Here's how the part is built. I have some questions about the finished solid (model axes, mm). Coordinates: 2 decimals unless noted, no trailing zeros. Write each loop counter-clockwise with the first axis right and the second up, starting at its lowest first coordinate (ties: lowest second). Pieces come first, ordered by that corner, then holes. Notation, with made-up numbers: M 15,89.5 L 27,89.5 A7 cw 27,96.5 Z; hole C 24.25,-26 d11. An arc over 180 degrees is marked long. Use one line per item in the form item = value. Start each with the question number.
1. I want a section at A-A, the plane z = 125.5. List the corners of the cut face in (x, y) for me.
2. Please list where these lines run through material, in increasing order: line 1 along X through (y, z) = (7.25, 121); line 2 along Z through (x, y) = (26, 8.25); line 3 along X through (y, z) = (8.75, 178). Write a range as [from, to].
3. I'm going to push flat-ended pins straight in: pin 1 Ø3 at (y, z) = (4, 230.5) entering from -X; pin 2 Ø6 at (x, z) = (83.5, 111) entering from -Y; pin 3 Ø3 at (x, y) = (201.5, 5.5) entering from -Z. Where does each tip first touch, or does it pass through?
4. I want a section at B-B, the plane z = 212. List the corners of the cut face in (x, y) for me.
5. I want a section at C-C, the plane y = 2. Count the separate pieces of the cut face and the enclosed holes in it, plus the area to 3 significant figures.
from build123d import *

# Parameters (mm, degrees)
SKETCH_1_R      = 3.519137415
SKETCH_1_R_2    = 4.021871331
SKETCH_1_R_3    = 4.053170413
SKETCH_1_R_4    = 3.845688718
SKETCH_1_R_5    = 4
EXTRUDE_1_DEPTH = 10


with BuildPart() as part:
    # 草图1 → 凸台-拉伸1 (new body)
    with BuildSketch(Plane(origin=(0, 0, 0), x_dir=(1, 0, 0), z_dir=(0, 1, 0))):
        Polygon((0, -50), (75, -50), (75, 0), (175, 0), (175, -50), (250, -50), (250, -200), (175, -200), (175, -250), (75, -250), (75, -200), (0, -200), align=None)
        with Locations(Location((140.533556543, -125.014564911, 0), (0, 0, 270))):
            Circle(SKETCH_1_R, mode=Mode.SUBTRACT)
        with Locations(Location((121.008156214, -98.872401259, 0), (0, 0, 270))):
            Circle(SKETCH_1_R_2, mode=Mode.SUBTRACT)
        with Locations(Location((121.008156214, -150.151260731, 0), (0, 0, 270))):
            Circle(SKETCH_1_R_3, mode=Mode.SUBTRACT)
        with Locations(Location((99.599362347, -125.014564911, 0), (0, 0, 270))):
            Circle(SKETCH_1_R_4, mode=Mode.SUBTRACT)
        with Locations(Location((85.515139111, -8.883030225, 0), (0, 0, 270))):
            Circle(SKETCH_1_R_5, mode=Mode.SUBTRACT)
        with Locations(Location((85.515139111, -30.50058863, 0), (0, 0, 270))):
            Circle(SKETCH_1_R_5, mode=Mode.SUBTRACT)
        with Locations(Location((107.349135631, -8.883030225, 0), (0, 0, 270))):
            Circle(SKETCH_1_R_5, mode=Mode.SUBTRACT)
        with Locations(Location((107.349135631, -30.50058863, 0), (0, 0, 270))):
            Circle(SKETCH_1_R_5, mode=Mode.SUBTRACT)
        with Locations(Location((146.396218991, -8.883030225, 0), (0, 0, 270))):
            Circle(SKETCH_1_R_5, mode=Mode.SUBTRACT)
        with Locations(Location((166.756942605, -8.883030225, 0), (0, 0, 270))):
            Circle(SKETCH_1_R_5, mode=Mode.SUBTRACT)
        with Locations(Location((146.396218991, -30.50058863, 0), (0, 0, 270))):
            Circle(SKETCH_1_R_5, mode=Mode.SUBTRACT)
        with Locations(Location((166.756942605, -30.50058863, 0), (0, 0, 270))):
            Circle(SKETCH_1_R_5, mode=Mode.SUBTRACT)
        with Locations(Location((85.515139111, -237.626962183, 0), (0, 0, 270))):
            Circle(SKETCH_1_R_5, mode=Mode.SUBTRACT)
        with Locations(Location((85.515139111, -212.99300028, 0), (0, 0, 270))):
            Circle(SKETCH_1_R_5, mode=Mode.SUBTRACT)
        with Locations(Location((107.217902356, -212.99300028, 0), (0, 0, 270))):
            Circle(SKETCH_1_R_5, mode=Mode.SUBTRACT)
        with Locations(Location((107.217902356, -237.626962183, 0), (0, 0, 270))):
            Circle(SKETCH_1_R_5, mode=Mode.SUBTRACT)
        with Locations(Location((162.537022604, -212.99300028, 0), (0, 0, 270))):
            Circle(SKETCH_1_R_5, mode=Mode.SUBTRACT)
        with Locations(Location((162.537022604, -237.626962183, 0), (0, 0, 270))):
            Circle(SKETCH_1_R_5, mode=Mode.SUBTRACT)
        with Locations(Location((140.533556543, -212.99300028, 0), (0, 0, 270))):
            Circle(SKETCH_1_R_5, mode=Mode.SUBTRACT)
        with Locations(Location((140.533556543, -237.626962183, 0), (0, 0, 270))):
            Circle(SKETCH_1_R_5, mode=Mode.SUBTRACT)
        with Locations(Location((9.903960691, -59.156421864, 0), (0, 0, 270))):
            Circle(SKETCH_1_R_5, mode=Mode.SUBTRACT)
        with Locations(Location((242.167030064, -59.156421864, 0), (0, 0, 270))):
            Circle(SKETCH_1_R_5, mode=Mode.SUBTRACT)
        with Locations(Location((242.167030064, -187.85630446, 0), (0, 0, 270))):
            Circle(SKETCH_1_R_5, mode=Mode.SUBTRACT)
        with Locations(Location((204.964720251, -59.156421864, 0), (0, 0, 270))):
            Circle(SKETCH_1_R_5, mode=Mode.SUBTRACT)
        with Locations(Location((204.964720251, -187.85630446, 0), (0, 0, 270))):
            Circle(SKETCH_1_R_5, mode=Mode.SUBTRACT)
        with Locations(Location((9.903960691, -187.85630446, 0), (0, 0, 270))):
            Circle(SKETCH_1_R_5, mode=Mode.SUBTRACT)
        with Locations(Location((43.587133089, -59.156421864, 0), (0, 0, 270))):
            Circle(SKETCH_1_R_5, mode=Mode.SUBTRACT)
        with Locations(Location((43.587133089, -187.85630446, 0), (0, 0, 270))):
            Circle(SKETCH_1_R_5, mode=Mode.SUBTRACT)
        with Locations(Location((69.226562825, -59.156421864, 0), (0, 0, 270))):
            Circle(SKETCH_1_R_5, mode=Mode.SUBTRACT)
        with Locations(Location((69.226562825, -187.85630446, 0), (0, 0, 270))):
            Circle(SKETCH_1_R_5, mode=Mode.SUBTRACT)
        with Locations(Location((179.828024432, -59.156421864, 0), (0, 0, 270))):
            Circle(SKETCH_1_R_5, mode=Mode.SUBTRACT)
        with Locations(Location((179.828024432, -187.85630446, 0), (0, 0, 270))):
            Circle(SKETCH_1_R_5, mode=Mode.SUBTRACT)
        with BuildLine():
            Line((31.521519096, -110.938015252), (31.521519096, -139.09111457))
            ThreePointArc((31.521519096, -139.09111457), (26.494179932, -144.118453734), (21.466840768, -139.09111457))
            Line((21.466840768, -139.09111457), (21.466840768, -110.938015252))
            ThreePointArc((21.466840768, -110.938015252), (26.494179932, -105.910676088), (31.521519096, -110.938015252))
        make_face(mode=Mode.SUBTRACT)
        with BuildLine():
            Line((31.521519096, -59.156421864), (31.521519096, -88.314989015))
            ThreePointArc((31.521519096, -88.314989015), (26.494179932, -93.342328179), (21.466840768, -88.314989015))
            Line((21.466840768, -88.314989015), (21.466840768, -59.156421864))
            ThreePointArc((21.466840768, -59.156421864), (26.494179932, -54.1290827), (31.521519096, -59.156421864))
        make_face(mode=Mode.SUBTRACT)
        with BuildLine():
            Line((21.969574685, -193.889111457), (21.969574685, -162.216874724))
            ThreePointArc((21.969574685, -162.216874724), (26.494179932, -157.692269477), (31.01878518, -162.216874724))
            Line((31.01878518, -162.216874724), (31.01878518, -193.889111457))
            ThreePointArc((31.01878518, -193.889111457), (26.494179932, -198.413716704), (21.969574685, -193.889111457))
        make_face(mode=Mode.SUBTRACT)
        with BuildLine():
            Line((232.615085653, -59.156421864), (232.615085653, -88.314989015))
            ThreePointArc((232.615085653, -88.314989015), (227.085012572, -93.845062095), (221.554939492, -88.314989015))
            Line((221.554939492, -88.314989015), (221.554939492, -59.156421864))
            ThreePointArc((221.554939492, -59.156421864), (227.085012572, -53.626348784), (232.615085653, -59.156421864))
        make_face(mode=Mode.SUBTRACT)
        with BuildLine():
            Line((232.615085653, -110.938015252), (232.615085653, -139.09111457))
            ThreePointArc((232.615085653, -139.09111457), (227.085012572, -144.621187651), (221.554939492, -139.09111457))
            Line((221.554939492, -139.09111457), (221.554939492, -110.938015252))
            ThreePointArc((221.554939492, -110.938015252), (227.085012572, -105.407942172), (232.615085653, -110.938015252))
        make_face(mode=Mode.SUBTRACT)
        with BuildLine():
            Line((232.112351736, -162.216874724), (232.112351736, -193.889111457))
            ThreePointArc((232.112351736, -193.889111457), (227.085012572, -198.916450621), (222.057673408, -193.889111457))
            Line((222.057673408, -193.889111457), (222.057673408, -162.216874724))
            ThreePointArc((222.057673408, -162.216874724), (227.085012572, -157.18953556), (232.112351736, -162.216874724))
        make_face(mode=Mode.SUBTRACT)
        with BuildLine():
            Line((86.319515983, -98.872401259), (86.319515983, -158.195003393))
            ThreePointArc((86.319515983, -158.195003393), (79.281241153, -165.233278223), (72.242966324, -158.195003393))
            Line((72.242966324, -158.195003393), (72.242966324, -98.872401259))
            ThreePointArc((72.242966324, -98.872401259), (79.281241153, -91.834126429), (86.319515983, -98.872401259))
        make_face(mode=Mode.SUBTRACT)
        with BuildLine():
            Line((174.297951351, -98.872401259), (174.297951351, -158.195003393))
            ThreePointArc((174.297951351, -158.195003393), (166.756942605, -165.736012139), (159.215933859, -158.195003393))
            Line((159.215933859, -158.195003393), (159.215933859, -98.872401259))
            ThreePointArc((159.215933859, -98.872401259), (166.756942605, -91.331392513), (174.297951351, -98.872401259))
        make_face(mode=Mode.SUBTRACT)
        with BuildLine():
            Line((94.951197402, -63.772444805), (113.552352308, -104.493892032))
            ThreePointArc((113.552352308, -104.493892032), (111.867528025, -109.012284427), (107.349135631, -107.327460144))
            Line((107.349135631, -107.327460144), (88.747980724, -66.606012917))
            ThreePointArc((88.747980724, -66.606012917), (90.432805007, -62.087620522), (94.951197402, -63.772444805))
        make_face(mode=Mode.SUBTRACT)
        with BuildLine():
            Line((162.851897535, -65.984783395), (137.212467799, -108.123014678))
            ThreePointArc((137.212467799, -108.123014678), (131.364165534, -109.546639764), (129.940540448, -103.698337499))
            Line((129.940540448, -103.698337499), (155.579970184, -61.560106215))
            ThreePointArc((155.579970184, -61.560106215), (161.428272449, -60.136481129), (162.851897535, -65.984783395))
        make_face(mode=Mode.SUBTRACT)
        with BuildLine():
            Line((85.515139111, -171.644415429), (107.217902356, -138.787064009))
            ThreePointArc((107.217902356, -138.787064009), (112.586083341, -137.689561768), (113.683585583, -143.057742753))
            Line((113.683585583, -143.057742753), (91.980822338, -175.915094173))
            ThreePointArc((91.980822338, -175.915094173), (86.612641352, -177.012596415), (85.515139111, -171.644415429))
        make_face(mode=Mode.SUBTRACT)
        with BuildLine():
            Line((140.533556543, -138.95433705), (162.537022604, -176.084926759))
            ThreePointArc((162.537022604, -176.084926759), (161.184000191, -181.374081835), (155.894845115, -180.021059422))
            Line((155.894845115, -180.021059422), (133.891379055, -142.890469712))
            ThreePointArc((133.891379055, -142.890469712), (135.244401467, -137.601314637), (140.533556543, -138.95433705))
        make_face(mode=Mode.SUBTRACT)
    extrude(amount=EXTRUDE_1_DEPTH)


solid = part.part
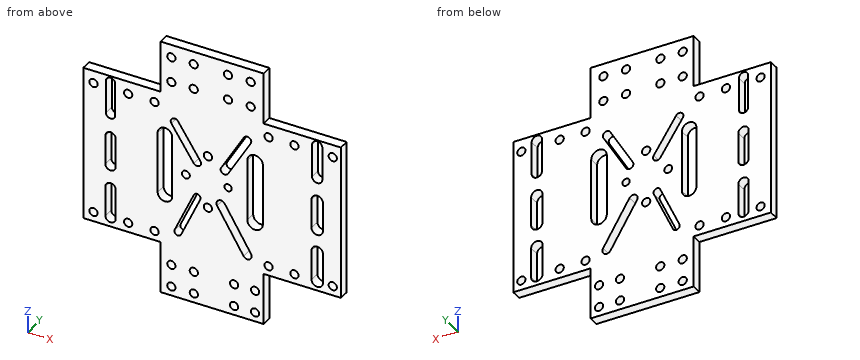
Answer list:
q1.outline = M 0,0 L 21.47,0 L 21.47,10 L 0,10 Z; M 31.52,0 L 72.24,0 L 72.24,10 L 31.52,10 Z; M 86.32,0 L 95.78,0 L 95.78,10 L 86.32,10 Z; M 103.41,0 L 137.05,0 L 137.05,10 L 103.41,10 Z; M 144.02,0 L 159.22,0 L 159.22,10 L 144.02,10 Z; M 174.3,0 L 221.55,0 L 221.55,10 L 174.3,10 Z; M 232.62,0 L 250,0 L 250,10 L 232.62,10 Z
q2.line_1 = [0, 21.47], [31.52, 72.24], [86.32, 159.22], [174.3, 221.55], [232.62, 250]
q2.line_2 = [50, 54.15], [93.32, 105.94], [144.09, 157.72], [198.39, 200]
q2.line_3 = [0, 21.97], [31.02, 154.7], [163.08, 222.06], [232.11, 250]
q3.pin_1 = 75
q3.pin_2 = 0
q3.pin_3 = 50
q4.outline = M 75,0 L 81.64,0 L 81.64,10 L 75,10 Z; M 89.39,0 L 103.34,0 L 103.34,10 L 89.39,10 Z; M 111.09,0 L 136.66,0 L 136.66,10 L 111.09,10 Z; M 144.41,0 L 158.66,0 L 158.66,10 L 144.41,10 Z; M 166.41,0 L 175,0 L 175,10 L 166.41,10 Z
q5.separate_pieces = 1
q5.enclosed_holes = 44
q5.area = 40,000 mm²
